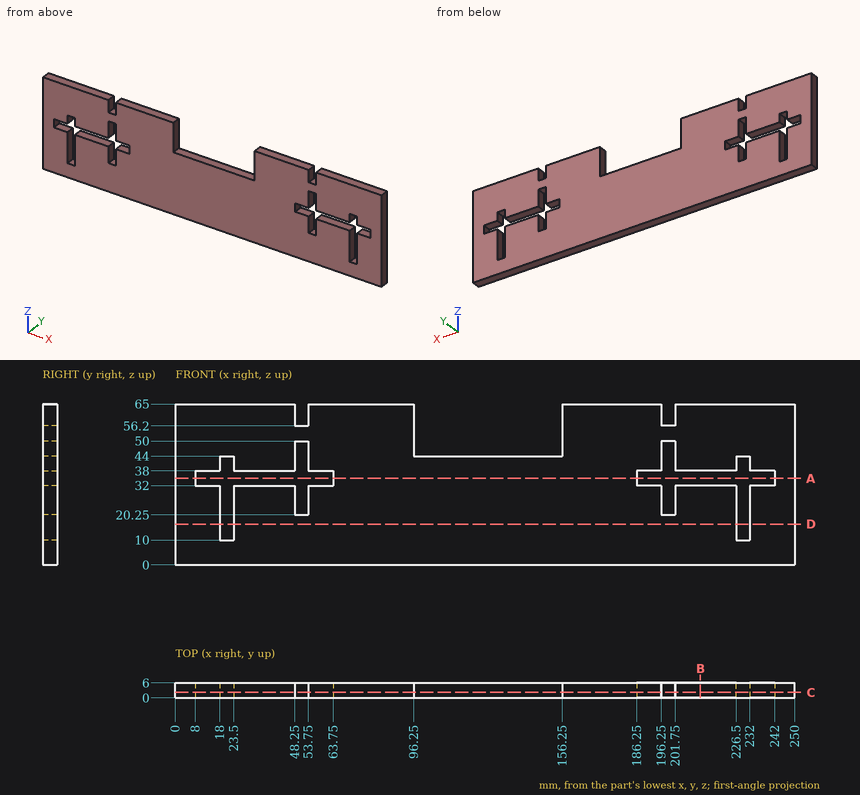
Part print with two shaded views. Sizes in mm from the minimum x, y, z corner. Round coordinates to 2 decimals unless told otherwise and drop trailing zeros. Loops run counter-clockwise (first coordinate to the right, second up) from the corner with the lowest first, then second, coordinate; pieces in that order, holes last. Notation, with made-up numbers: M 40.5,-35 L 76.5,-35 A20 cw 76.5,-18 Z; hole C -12.5,24.25 d6. An arc over 180 degrees is marked long. Return JSON: item names as keys, results as strings. Group by question number.
(1) Saw through at B-B, the plane x = 212. List the corners of the cut face in (y, z).
(2) Wall check: probe 1 along X at (y, z) = (5.3, 42.5); probe 2 along X at (y, z) = (5.05, 46); probe 3 along X at (y, z) = (5.5, 37.5). Give the ranges that are in metal, low to high. Write a range as [from, to].
(3) Saw through at D-D, the plane z = 16.5. List the corners of the cut face in (x, y).
(4) Saw through at C-C, the plane y = 2.2. Give the number of separate pieces and of enclosed holes in the cut face, and give its area (3 significant figures).
(5) Saw through at A-A, the plane z = 35. List the corners of the cut face in (x, y).
Answer list:
{
 "1": {"outline": "M 0,0 L 6,0 L 6,32 L 0,32 Z; M 0,38 L 6,38 L 6,65 L 0,65 Z"},
 "2": {"probe 1": "[0, 18], [23.5, 48.25], [53.75, 196.25], [201.75, 226.5], [232, 250]", "probe 2": "[0, 48.25], [53.75, 96.25], [156.25, 196.25], [201.75, 250]", "probe 3": "[0, 8], [63.75, 186.25], [242, 250]"},
 "3": {"outline": "M 0,0 L 18,0 L 18,6 L 0,6 Z; M 23.5,0 L 226.5,0 L 226.5,6 L 23.5,6 Z; M 232,0 L 250,0 L 250,6 L 232,6 Z"},
 "4": {"separate pieces": "1", "enclosed holes": "2", "area": "13,700 mm2"},
 "5": {"outline": "M 0,0 L 8,0 L 8,6 L 0,6 Z; M 63.75,0 L 186.25,0 L 186.25,6 L 63.75,6 Z; M 242,0 L 250,0 L 250,6 L 242,6 Z"}
}
